from build123d import *

# Parameters (mm, degrees)
BASE_FLANGE1_DEPTH = 2.286
SKETCH6_R          = 6.35
CUT_EXTRUDE1_DEPTH = 275.752517361
EDGE_FLANGE1_DEPTH = 152.4
FILLET1_R          = 6.35
EDGE_FLANGE2_DEPTH = 127
UNFOLD1_START      = 12.7
UNFOLD1_DEPTH      = 127
UNFOLD1_2_DEPTH    = 127
SKETCH15_W         = 25.4
SKETCH15_H         = 152.4
SKETCH15_H_2       = 57.15
CUT_EXTRUDE2_DEPTH = 2.54
FOLD1_START        = 38.1
FOLD1_DEPTH        = 101.6
FOLD1_2_DEPTH      = 76.2
FOLD1_START_2      = 114.3
FOLD1_3_DEPTH      = 25.4
FILLET2_R          = 3.175
SKETCH16_W         = 15.875
SKETCH16_H         = 203.2
CUT_EXTRUDE3_DEPTH = 337.68309673
SKETCH17_R         = 2.413
CUT_EXTRUDE4_DEPTH = 337.68309673
SKETCH18_R         = 2.413
CUT_EXTRUDE5_DEPTH = 2.54


# Read off the part's stored shape, not the designer's step: Unfold1, Fold1
# Sheet-metal steps are written as plain solids
with BuildPart() as part:
    # Sketch1 → Base-Flange1 (new body)
    with BuildSketch(Plane.XY):
        Polygon((139.7, 94.742), (152.4, 94.742), (152.4, 0), (0, 0), (0, 94.742), (12.7, 94.742), (12.7, 228.6), (139.7, 228.6), align=None)
    extrude(amount=-BASE_FLANGE1_DEPTH)

    # Sketch6 → Cut-Extrude1 (cut, through all)
    with BuildSketch(Plane.XY):
        with Locations((27.051, 69.85)):
            Circle(SKETCH6_R)
    extrude(amount=-CUT_EXTRUDE1_DEPTH, mode=Mode.SUBTRACT)

    # Edge-Flange1 section (across the edge) → Edge-Flange1 (add)
    with BuildSketch(Plane(origin=(152.4, -14.136010759, -2.286), x_dir=(0, 0.7431448254773909, -0.6691306063588619), z_dir=(-1, 0, 0))):
        with BuildLine():
            Line((-2.286, 14.136010759), (-2.286, 107.440207225))
            Line((-2.286, 107.440207225), (0, 107.440207225))
            Line((0, 107.440207225), (0, 14.136010759))
            ThreePointArc((0, 14.136010759), (2.74493172, 1.222122341), (10.505103248, -9.45883745))
            Line((10.505103248, -9.45883745), (8.975470682, -11.157666521))
            ThreePointArc((8.975470682, -11.157666521), (0.656566804, 0.292322375), (-2.286, 14.136010759))
        make_face()
    extrude(amount=EDGE_FLANGE1_DEPTH)

    # Fillet1
    fillet1_edges = [part.edges().sort_by_distance(p)[0] for p in [
        (152.4, -86.876956302, -81.364817765),
        (0, -86.876956302, -81.364817765),
    ]]
    fillet(fillet1_edges, radius=FILLET1_R)

    # Edge-Flange2 section (across the edge) → Edge-Flange2 (add)
    with BuildSketch(Plane(origin=(12.7, 246.930871047, -2.286), x_dir=(0, -0.8660254037844364, -0.5000000000000041), z_dir=(1, 0, 0))):
        with BuildLine():
            Line((-2.286, 18.330871047), (-2.286, 79.706177285))
            Line((-2.286, 79.706177285), (0, 79.706177285))
            Line((0, 79.706177285), (0, 18.330871047))
            ThreePointArc((0, 18.330871047), (4.25369343, 2.455871047), (15.875, -9.165435523))
            Line((15.875, -9.165435523), (14.732, -11.145169596))
            ThreePointArc((14.732, -11.145169596), (2.273959357, 1.312871047), (-2.286, 18.330871047))
        make_face()
    extrude(amount=EDGE_FLANGE2_DEPTH)

    # Unfold1 outline → Unfold1 (cut)
    with BuildSketch(Plane.YZ.offset(UNFOLD1_START)):
        with BuildLine():
            Line((240.863229427, -2.286), (228.6, -2.286))
            ThreePointArc((228.6, -2.286), (244.475, -6.53969343), (256.09630657, -18.161))
            Line((256.09630657, -18.161), (286.783959689, -71.313574367))
            Line((286.783959689, -71.313574367), (288.763693762, -70.170574367))
            Line((288.763693762, -70.170574367), (258.076040643, -17.018))
            ThreePointArc((258.076040643, -17.018), (250.731417092, -8.177738777), (240.863229427, -2.286))
        make_face()
    extrude(amount=UNFOLD1_DEPTH, mode=Mode.SUBTRACT)

    # Unfold1 2 outline → Unfold1 2 (add)
    with BuildSketch(Plane.YZ.offset(UNFOLD1_START)):
        with BuildLine():
            ThreePointArc((228.6, 0), (234.837238812, -0.576380337), (240.863229427, -2.286))
            Line((240.863229427, -2.286), (324.420775289, -2.286))
            Line((324.420775289, -2.286), (324.420775289, 0))
            Line((324.420775289, 0), (228.6, 0))
        make_face()
    extrude(amount=UNFOLD1_2_DEPTH)

    # Sketch15 → Cut-Extrude2 (cut)
    with BuildSketch(Plane.XY):
        with Locations((25.4, 248.220775289)):
            Rectangle(SKETCH15_W, SKETCH15_H)
        with Locations((127, 295.845775289)):
            Rectangle(SKETCH15_W, SKETCH15_H_2)
    extrude(amount=-CUT_EXTRUDE2_DEPTH, mode=Mode.SUBTRACT)

    # Fold1 outline → Fold1 (cut)
    with BuildSketch(Plane.YZ.offset(FOLD1_START)):
        with BuildLine():
            ThreePointArc((228.6, 0), (234.837238812, -0.576380337), (240.863229427, -2.286))
            Line((240.863229427, -2.286), (324.420775289, -2.286))
            Line((324.420775289, -2.286), (324.420775289, 0))
            Line((324.420775289, 0), (228.6, 0))
        make_face()
    extrude(amount=FOLD1_DEPTH, mode=Mode.SUBTRACT)

    # Fold1 2 outline → Fold1 2 (add)
    with BuildSketch(Plane.YZ.offset(FOLD1_START)):
        with BuildLine():
            ThreePointArc((228.6, -2.286), (244.475, -6.53969343), (256.09630657, -18.161))
            Line((256.09630657, -18.161), (286.783959689, -71.313574367))
            Line((286.783959689, -71.313574367), (288.763693762, -70.170574367))
            Line((288.763693762, -70.170574367), (258.076040643, -17.018))
            ThreePointArc((258.076040643, -17.018), (250.731417092, -8.177738777), (240.863229427, -2.286))
            Line((240.863229427, -2.286), (228.6, -2.286))
        make_face()
    extrude(amount=FOLD1_2_DEPTH)

    # Fold1 3 outline → Fold1 3 (add)
    with BuildSketch(Plane.YZ.offset(FOLD1_START_2)):
        with BuildLine():
            ThreePointArc((228.6, -2.286), (244.475, -6.53969343), (256.09630657, -18.161))
            Line((256.09630657, -18.161), (258.208959689, -21.820222541))
            Line((258.208959689, -21.820222541), (260.188693762, -20.677222541))
            Line((260.188693762, -20.677222541), (258.076040643, -17.018))
            ThreePointArc((258.076040643, -17.018), (250.731417092, -8.177738777), (240.863229427, -2.286))
            Line((240.863229427, -2.286), (228.6, -2.286))
        make_face()
    extrude(amount=FOLD1_3_DEPTH)

    # Fillet2
    fillet2_edges = [part.edges().sort_by_distance(p)[0] for p in [
        (38.1, 172.020775289, -1.143),
        (114.3, 259.198826725, -21.248722541),
    ]]
    fillet(fillet2_edges, radius=FILLET2_R)

    # Sketch16 → Cut-Extrude3 (cut, through all)
    with BuildSketch(Plane.XY):
        with Locations((76.04125, 298.45)):
            Rectangle(SKETCH16_W, SKETCH16_H)
    extrude(amount=-CUT_EXTRUDE3_DEPTH, mode=Mode.SUBTRACT)

    # Sketch17 → Cut-Extrude4 (cut, through all)
    with BuildSketch(Plane.XY):
        with Locations((6.35, 85.217)):
            Circle(SKETCH17_R)
        with Locations((6.35, 47.117)):
            Circle(SKETCH17_R)
        with Locations((6.35, 9.017)):
            Circle(SKETCH17_R)
        with Locations((146.05, 47.117)):
            Circle(SKETCH17_R)
        with Locations((146.05, 9.017)):
            Circle(SKETCH17_R)
        with Locations((146.05, 85.217)):
            Circle(SKETCH17_R)
    extrude(amount=-CUT_EXTRUDE4_DEPTH, mode=Mode.SUBTRACT)

    # Sketch18 → Cut-Extrude5 (cut)
    with BuildSketch(Plane(origin=(0, -8.368903665, 7.535394706), x_dir=(1, 0, 0), z_dir=(0, -0.7431448254773909, 0.6691306063588619))):
        with Locations(Location((6.35, -37.99367728, 0), (0, 0, 270))):
            Circle(SKETCH18_R)
        with Locations(Location((146.05, -37.99367728, 0), (0, 0, 270))):
            Circle(SKETCH18_R)
    extrude(amount=-CUT_EXTRUDE5_DEPTH, mode=Mode.SUBTRACT)


solid = part.part
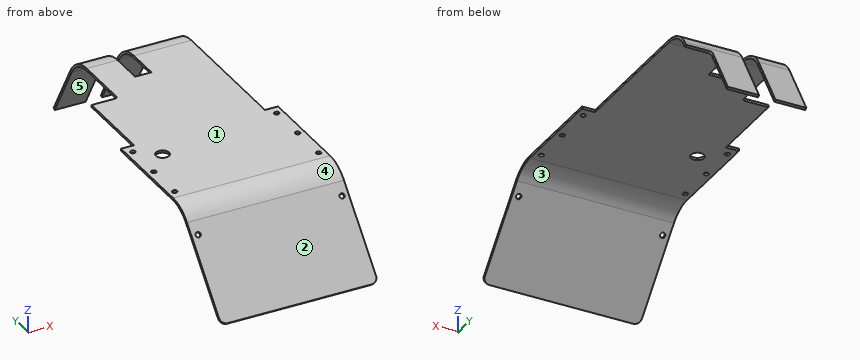
Geometry: final body of the model. Coordinates: model frame, mm. Face numbers are marked on the shaded views. A direction names the side the tool comes from. Round coordinates to 2 decimals unless told otherwise and drop trailing zeros. Loops run counter-clockwise (first coordinate to the right, second up) from the corner with the lowest first, then second, coordinate; pieces in that order, holes last. Notation, with made-up numbers: M 74.25,-37 L 118.25,-37 A21 cw 118.25,-19 Z; hole C 38,16.5 d8. An arc over 180 degrees is marked long. Put each result on its own line as item: value. Start each with the question number.
(1) Set-up query: the marked faces 4 and 5. Return all of +Z, -Z, +X, -X, +Y, -Y with unobstructed straight access to the full face (end or side cutting, diameter ignored); none if empty.
(2) Contact query for flat-ended pins moving along their axis: pin 1 Ø5 at (x, z) = (100, -72.5) entering from -Y; pin 2 Ø5.5 at (x, y) = (146.05, 85.217) entering from -Z; pin 3 Ø1.8 at (x, z) = (4.5, -1.5) entering from +Y. Output: stop coordinate, or through.
(3) Section query A-A (y = 69.85). Return loops of the section in (x, z).
(4) Draft query along Y for the marked faces 1, 2 and 3. Return one class per face: +Y half, -Y half, draft (parallel to the pull), parting line (faces both ways), or undercut.
(5) Section query B-B (x = 107.5). Return loops of the section in (y, z).
(6) Section query C-C (z = -56). Return loops of the section in (x, y), then the cut area to 3 significant figures.
(7) Material intervals for line 1 along Y through (x, z) = (64.5, -10); line 2 along Y through (x, z) = (115, -5); line 3 along Z through (x, y) = (105, 19), sorted ascending. Write a range as [from, to].
Findings below:
1. face 4: +Z, +X, -X, -Y
1. face 5: -Z, +X, -X
2. pin 1: stops at y = -82.68
2. pin 2: stops at z = -2.29
2. pin 3: stops at y = 94.74
3. outline: M 0,-2.29 L 20.7,-2.29 L 20.7,0 L 0,0 Z; M 33.4,-2.29 L 152.4,-2.29 L 152.4,0 L 33.4,0 Z
4. face 1: draft
4. face 2: -Y half
4. face 3: undercut
5. outline: M -87.73,-80.6 L -86.03,-82.13 L -23.59,-12.79 A31.75 cw 0,-2.29 L 228.6,-2.29 A31.75 cw 256.1,-18.16 L 286.78,-71.31 L 288.76,-70.17 L 258.08,-17.02 A34.04 ccw 228.6,0 L 0,0 A34.04 ccw -25.29,-11.26 Z
6. outline: M 0,-65.58 L 152.4,-65.58 L 152.4,-62.5 L 0,-62.5 Z; M 38.1,277.94 L 68.1,277.94 L 68.1,280.58 L 38.1,280.58 Z; M 83.98,277.94 L 114.3,277.94 L 114.3,280.58 L 83.98,280.58 Z
6. area: 628 mm2
7. line 1: y = [-24.1, -20.74], [249.34, 252.7]
7. line 2: y = [-17.76, -12.84], [241.44, 246.36]
7. line 3: z = [-2.29, 0]
